Source: CAD feature listing. Evaluate the final solid. Frame: model axes, mm. Face numbers are marked on the shaded views. A direction names the side the tool comes from. Give positions to 0.01 mm unless a question says otherwise; leave off trailing zeros. Write each loop counter-clockwise with the first axis right and the second up, starting at its lowest first coordinate (ties: lowest second). Pieces come first, ordered by that corner, then holes.
```python
from build123d import *

# Parameters (mm, degrees)
F1_DEPTH = 62.5
F2_DEPTH = 25
F3_DEPTH = 10
F0_W     = 25.4
F0_H     = 19.05
F4_DEPTH = 25
F6_R     = 6.3


with BuildPart() as f1:
    # F0 (on Front) → F1 (new body, symmetric)
    with BuildSketch(Plane.XZ):
        Polygon((22.225, 9.525), (-41.275, 9.525), (-41.275, -9.525), (41.275, -9.525), (41.275, 9.525), align=None)
    extrude(amount=F1_DEPTH, both=True)

    # F0 (on Front) → F2 (join, symmetric)
    with BuildSketch(Plane.XZ):
        with BuildLine():
            Line((22.225, 27), (22.225, 9.525))
            Line((22.225, 9.525), (41.275, 9.525))
            Line((41.275, 9.525), (41.275, 27))
            ThreePointArc((41.275, 27), (45.9246798487, 38.2253201513), (57.15, 42.875))
            Line((57.15, 42.875), (60.325, 42.875))
            Line((60.325, 42.875), (60.325, 61.925))
            Line((60.325, 61.925), (57.15, 61.925))
            add(Edge.make_bspline(
                [(56.3095148164, 61.9148852161), (56.5902291642, 61.9192274348), (56.8703973727, 61.9226005748), (57.15, 61.925)],
                knots=[110.7716747291, 110.7716747291, 110.7716747291, 110.7716747291, 111.5044421761, 111.5044421761, 111.5044421761, 111.5044421761], degree=3))
            ThreePointArc((56.3095148164, 61.9148852161), (32.1589058859, 51.3967383062), (22.225, 27))
        make_face()
    extrude(amount=F2_DEPTH, both=True)

    # F0 (on Front) → F3 (join, symmetric)
    with BuildSketch(Plane.XZ):
        with BuildLine():
            add(Edge.make_bspline(
                [(-41.275, 9.525), (-41.0414624957, 38.4566380676), (13.8742257665, 61.2584766517), (56.3095148164, 61.9148852161)],
                knots=[0, 0, 0, 0, 110.7716747291, 110.7716747291, 110.7716747291, 110.7716747291], degree=3))
            Line((-41.275, 9.525), (22.225, 9.525))
            Line((22.225, 9.525), (22.225, 27))
            ThreePointArc((22.225, 27), (32.1589058859, 51.3967383062), (56.3095148164, 61.9148852161))
        make_face()
    extrude(amount=F3_DEPTH, both=True)

    # F0 (on Front) → F4 (join, symmetric)
    with BuildSketch(Plane.XZ):
        with Locations((73.025, 52.4)):
            Rectangle(F0_W, F0_H)
    extrude(amount=F4_DEPTH, both=True)

    # F0 (on Front) → F5 (revolve)
    with BuildSketch(Plane.XZ):
        Polygon((85.725, 66.675), (85.725, 61.925), (85.725, 42.875), (85.725, 38.1), (111.125, 38.1), (111.125, 66.675), align=None)
    revolve(axis=Axis((85.725, 0, 52.3875), (0, 0, 1)))

    # F6
    f6_edges = [f1.edges().sort_by_distance(p)[0] for p in [
        (41.275, -62.5, 0),
        (-41.275, -62.5, 0),
        (41.275, 62.5, 0),
        (-41.275, 62.5, 0),
    ]]
    fillet(f6_edges, radius=F6_R)


solid = f1.part
```
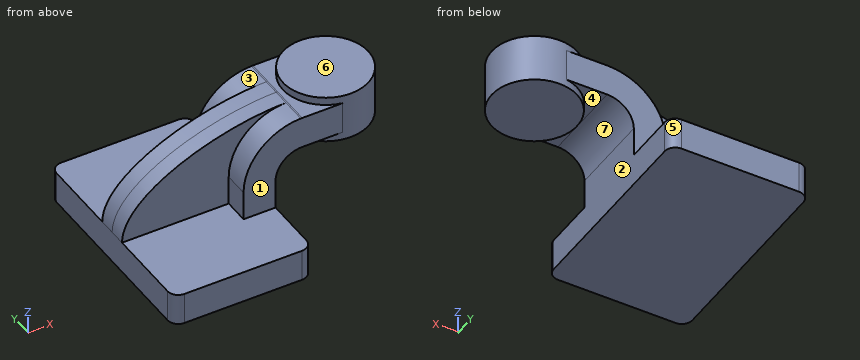
1. Access query for the marked faces 1, 2, 3 and 4. Directions: +Z, -Z, +X, -X, +Y, -Y. A direction counts if a zero-diameter tool reaches every point of the face in a straight line with its end or side. Return the directions, or none.
2. Cut plane B-B, the plane y = 48.5. Return the cut outline in (x, z) (3 decimals).
3. Cut plane A-A, the plane z = -2. Return the cut outline in (x, y) (3 decimals), then the cut area to 3 significant figures.
4. Contact query for flat-ended pins moving along their axis: P1, Ø12, axis at y = 29, z = 7.5, coming from the +X side (3 decimals); P2, Ø1.5, axis at y = 37, z = 10, coming from the -X side (3 decimals); P3, Ø12, axis at y = -18.5, z = 22, coming from the -X side (3 decimals); P4, Ø15.5, axis at x = 24.5, z = 48.5, coming from the +Y side. Output: stop coordinate, or through.
5. Cut plane C-C, the plane x = 83.5. Return the cut outline in (y, z) (3 decimals), then the cut area to 3 significant figures.
6. Line query: L1, parallel to Z at x = 33, y = 34 (3 decimals); L2, parallel to Z at x = 71.5, y = -14.5 (3 decimals); L3, parallel to X at y = 13.5, z = 40.5. Output: solid intervals per line, ascending.
7. Mould query, pull axis X, two halves, no side actions, for the marked faces 5, 6 and 7. Classes: +X half, -X half, draft (parallel to the pull), parting line (faces both ways), or undercut.
Response values:
1. face 1: +Z, -X, -Y
1. face 2: -Z, +X, +Y, -Y
1. face 3: +Z, -X, +Y
1. face 4: -Z
2. outline: (-41.275, -9.525) - (41.275, -9.525) - (41.275, 9.525) - (-41.275, 9.525) - close
3. outline: (-41.275, -56.2) arc R6.3 ccw to (-34.975, -62.5) - (34.975, -62.5) arc R6.3 ccw to (41.275, -56.2) - (41.275, 56.2) arc R6.3 ccw to (34.975, 62.5) - (-34.975, 62.5) arc R6.3 ccw to (-41.275, 56.2) - close
3. area: 10,300 mm2
4. P1: stops at x = 41.275
4. P2: stops at x = -41.275
4. P3: stops at x = 22.225
4. P4: stops at y = 25
5. outline: (-25.302, 38.1) - (25.302, 38.1) - (25.302, 66.675) - (-25.302, 66.675) - close
5. area: 1,450 mm2
6. L1: z = -9.525 to 9.525
6. L2: z = 38.1 to 66.675
6. L3: x = 24.94 to 48.8, 64.21 to 107.24
7. face 5: +X half
7. face 6: draft
7. face 7: undercut
